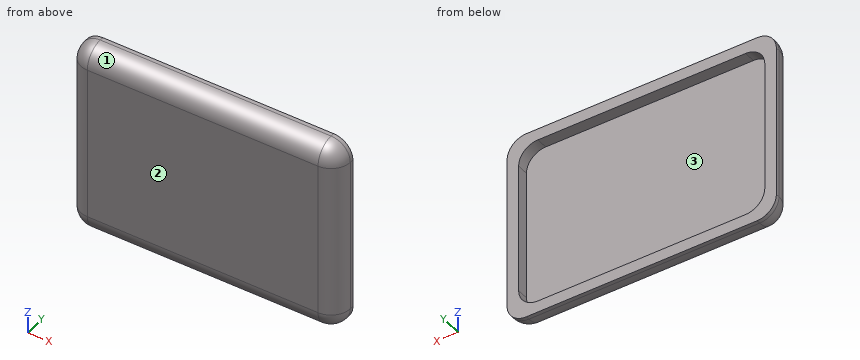
from build123d import *

# Parameters (mm, degrees)
SKETCH1_W           = 70
SKETCH1_H           = 50
BOSS_EXTRUDE1_DEPTH = 6
SHELL1_T            = -3
FILLET1_R           = 5
FILLET2_R           = 5
FILLET3_R           = 5
FILLET4_R           = 5
FILLET5_R           = 5
FILLET6_R           = 5
FILLET7_R           = 5
FILLET8_R           = 5
FILLET9_R           = 5


with BuildPart() as part:
    # Sketch1 → Boss-Extrude1 (new body)
    with BuildSketch(Plane(origin=(0, 0, 0), x_dir=(1, 0, 0), z_dir=(0, 1, 0))):
        Rectangle(SKETCH1_W, SKETCH1_H)
    extrude(amount=BOSS_EXTRUDE1_DEPTH)

    # Shell1
    shell1_openings = [part.faces().sort_by_distance(p)[0] for p in [
        (0, 6, 0),
    ]]
    offset(amount=SHELL1_T, openings=shell1_openings, kind=Kind.INTERSECTION)

    # Fillet1
    fillet1_edges = [part.edges().sort_by_distance(p)[0] for p in [
        (35, 3, 25),
    ]]
    fillet(fillet1_edges, radius=FILLET1_R)

    # Fillet2
    fillet2_edges = [part.edges().sort_by_distance(p)[0] for p in [
        (35, 3, -25),
    ]]
    fillet(fillet2_edges, radius=FILLET2_R)

    # Fillet3
    fillet3_edges = [part.edges().sort_by_distance(p)[0] for p in [
        (-35, 3, 25),
    ]]
    fillet(fillet3_edges, radius=FILLET3_R)

    # Fillet4
    fillet4_edges = [part.edges().sort_by_distance(p)[0] for p in [
        (-35, 3, -25),
    ]]
    fillet(fillet4_edges, radius=FILLET4_R)

    # Fillet5
    fillet5_edges = [part.edges().sort_by_distance(p)[0] for p in [
        (35, 0, 0),
        (0, 0, -25),
        (0, 0, 25),
        (-35, 0, 0),
    ]]
    fillet(fillet5_edges, radius=FILLET5_R)

    # Fillet6
    fillet6_edges = [part.edges().sort_by_distance(p)[0] for p in [
        (32, 4.5, 22),
    ]]
    fillet(fillet6_edges, radius=FILLET6_R)

    # Fillet7
    fillet7_edges = [part.edges().sort_by_distance(p)[0] for p in [
        (-32, 4.5, 22),
    ]]
    fillet(fillet7_edges, radius=FILLET7_R)

    # Fillet8
    fillet8_edges = [part.edges().sort_by_distance(p)[0] for p in [
        (-32, 4.5, -22),
    ]]
    fillet(fillet8_edges, radius=FILLET8_R)

    # Fillet9
    fillet9_edges = [part.edges().sort_by_distance(p)[0] for p in [
        (32, 4.5, -22),
    ]]
    fillet(fillet9_edges, radius=FILLET9_R)


solid = part.part
Design review of the part built by this model. Coordinates are the model's own, in mm. Face numbers are marked on the shaded views. Give positions to 0.01 mm unless a question says otherwise; leave off trailing zeros. Loops run counter-clockwise (first coordinate to the right, second up) from the corner with the lowest first, then second, coordinate; pieces in that order, holes last. Notation, with made-up numbers: (-13, -5.75) -> (-8, -5.75) arc R25 ccw to (-8, 22.25) -> close; hole circle Ø7 at (9, 18.5). An arc over 180 degrees is marked (long way). One line per question, with ' | ' between items. Start each with the question number.
(1) Insertion check: P1, Ø1, axis at y = 1, z = 0.5, coming from the +X side; P2, Ø13, axis at x = 11, z = 8, coming from the +Y side; P3, Ø3, axis at x = -22, y = 3, coming from the -Z side. Each pin has a flat end and moves straight along its axis. Give the tip position at first contact, or say it passes through.
(2) We need section C-C (x = 23). State the section outline as (y, z) points.
(3) We need section A-A (z = 10.5). State the section outline as (x, y) points.
(4) We need section B-B (y = 3.75). State the section outline as (x, z) points, and give its area (3 significant figures).
(5) For line 1 (X direction, y = 4.75, z = -4.5); line 2 (Z direction, x = 13, y = 4.75); line 3 (Y direction, x = 20, z = 3.5), list the stretches that pass through material, from the lowest coordinate up.
(6) Draft analysis for pull direction Z (two halves, no side actions). For the marked faces 1, 2 and 3, state which applies: +Z half, -Z half, draft (parallel to the pull), parting line (faces both ways), or undercut.
The answers:
1) P1: stops at x = 33.57 | P2: stops at y = 3 | P3: stops at z = -24.97
2) outline: (0, -20) arc R5 ccw to (5, -25) -> (6, -25) -> (6, -22) -> (3, -22) -> (3, 22) -> (6, 22) -> (6, 25) -> (5, 25) arc R5 ccw to (0, 20) -> close
3) outline: (-35, 5) arc R5 ccw to (-30, 0) -> (30, 0) arc R5 ccw to (35, 5) -> (35, 6) -> (32, 6) -> (32, 3) -> (-32, 3) -> (-32, 6) -> (-35, 6) -> close
4) outline: (-34.84, -20) arc R4.84 ccw to (-30, -24.84) -> (30, -24.84) arc R4.84 ccw to (34.84, -20) -> (34.84, 20) arc R4.84 ccw to (30, 24.84) -> (-30, 24.84) arc R4.84 ccw to (-34.84, 20) -> close; hole (-32, -17) arc R5 ccw to (-27, -22) -> (27, -22) arc R5 ccw to (32, -17) -> (32, 17) arc R5 ccw to (27, 22) -> (-27, 22) arc R5 ccw to (-32, 17) -> close | area: 647 mm^2
5) line 1: x = -34.99 to -32, 32 to 34.99 | line 2: z = -24.99 to -22, 22 to 24.99 | line 3: y = 0 to 3
6) face 1: +Z half | face 2: draft | face 3: undercut
